Source: CAD feature listing. Evaluate the final solid. Frame: model axes, mm. A direction names the side the tool comes from. Round coordinates to 2 decimals unless told otherwise and drop trailing zeros. Order: outer loops, then holes, each group sorted by start corner. A loop starts at its lowest first (then second) coordinate and runs counter-clockwise, first axis right, second up. Notation, with made-up numbers: (-2, -35.5) - (44, -35.5) arc R22 cw to (44, -28.5) - close; hole circle Ø2 at (-23.75, -37.75). An arc over 180 degrees is marked (long way). Use one line per item in the form item = value. Start each with the question number.
Q1. Cut plane D-D, the plane y = 5.75. Give the number of separate pieces and of enclosed holes in the cut face, and give its area (3 significant figures).
Q2. Ray query, line 1 (X direction, y = 7.75, z = 2.75); line 2 (Y direction, x = -22, z = 3); line 3 (X direction, y = 3.5, z = -12). Return the intervals inside material, ascending. Write a range as [from, to].
Q3. Draft query along X for faces 4 (the flat face through (-9, 3, -6.81)), 5 (the flat face through (-6.36, 3.94, 5.27)), 6 (the cylindrical face through (-21.13, 3.94, -10.83)). Return one class per face: released by +X, released by -X, zero draft, split by the parting line, or undercut.
Q4. Pin query (flat end, axial travel): pin 1 Ø2.5 at (x, y) = (-15, 3.5) entering from +Z; pin 2 Ø4 at (x, z) = (-7, -11.5) entering from -Y; pin 3 Ø0.8 at (x, y) = (0, 3.5) entering from +Z. Return the tip coordinate at first contact, or that it passes through.
Q5. Cut plane B-B, the plane x = 0. Return the cut outline in (y, z) (3 decimals).
Q6. Cut plane C-C, the plane y = 3.75. Return the cut outline in (x, z) (1 decimal), and give its area (3 significant figures).
Q7. Set-up query: faces 1 (the flat face through (0, 4, -0.925)), 2 (the flat face through (-10, 8, -6)), 3 (the flat face through (-20, 5.4, -3)). Return all of +Z, -Z, +X, -X, +Y, -Y with unobstructed straight access to the full face (end or side cutting, diameter ignored); none if empty.
Q8. Cut plane A-A, the plane z = -11. Return the cut outline in (x, y).
Autodesk Inventor part; units mm, degrees
ref_plane "YZ Plane" through (0, 0, 0) normal (1, 0, 0) x (0, 1, 0)
ref_plane "XZ Plane" through (0, 0, 0) normal (0, 1, 0) x (-1, 0, 0)
ref_plane "XY Plane" through (0, 0, 0) normal (0, 0, 1) x (1, 0, 0)
sketch "Sketch1" plane through (0, 0, 0) normal (0, 1, 0) x (-1, 0, 0)
  arc A0 (1.2748, -0.925) -> (-1.2748, -0.925) centre (0, 0) ccw
  line L0 (1.2748, -0.925) -> (-1.2748, -0.925)
  arc A1 (-0.8639, 3.4691) -> (-3.3372, -1.2821) centre (0, 0) ccw
  line L1 (-0.8639, 3.4691) -> (21.9124, 9.141)
  line L2 (-3.3372, -1.2821) -> (5.0806, -23.1927)
  arc A2 (5.0806, -23.1927) -> (21.9124, 9.141) centre (0, 0) ccw
  circle A3 centre (16.2426, 0) radius 4.075
  circle A4 centre (9.3164, -13.3052) radius 4.075
  circle A5 centre (16.2426, 0) radius 7.5 construction
  circle A6 centre (9.3164, -13.3052) radius 7.5 construction
  line L3 (0, 0) -> (16.2426, 0) construction
  line L4 (0, 0) -> (9.3164, -13.3052) construction
  line L5 (12.4926, -6.4952) -> (8.7426, 0)
  line L6 (8.7426, 0) -> (12.4926, 6.4952)
  line L7 (12.4926, 6.4952) -> (19.9926, 6.4952)
  line L8 (19.9926, 6.4952) -> (23.7426, 0)
  line L9 (23.7426, 0) -> (19.9926, -6.4952)
  line L10 (19.9926, -6.4952) -> (12.4926, -6.4952)
  line L11 (16.8164, -13.3052) -> (13.0664, -19.8004)
  line L12 (13.0664, -19.8004) -> (5.5664, -19.8004)
  line L13 (5.5664, -19.8004) -> (1.8164, -13.3052)
  line L14 (1.8164, -13.3052) -> (5.5664, -6.81)
  line L15 (5.5664, -6.81) -> (13.0664, -6.81)
  line L16 (13.0664, -6.81) -> (16.8164, -13.3052)
  dimension "d5" = 15
  dimension "d6" = 15
  dimension "d0" = 3.15
  dimension "d1" = 2.5
  dimension "d2" = 2
  dimension "d3" = 8.15
  dimension "d4" = 8.15
  dimension "d7" = 55
extrude "Extrusion1" add sketch "Sketch1" along normal blind 8 contours L9 L10 L5 L6 L7 L8 | L1 A2 L2 A1 | L11 L12 L13 L14 L15 L16
fillet "Fillet1" radius 8 2 edges at (-21.9124, 4, 9.141) (-5.0806, 4, -23.1927)
extrude "Extrusion2" cut sketch "Sketch1" along normal blind 5.4 contours L9 L10 L5 L6 L7 L8 | L11 L12 L13 L14 L15 L16
sketch "Sketch2" plane through (0, 0, 0) normal (0, -1, 0) x (1, 0, 0)
  arc A0 (-12.8561, -19.8004) -> (-6.2416, -19.8004) centre (-9.5488, -12.516) ccw
  line L0 (-6.2416, -19.8004) -> (-12.8561, -19.8004)
  arc A1 (-12.8561, -19.8004) -> (-6.2416, -19.8004) centre (-9.5488, -12.516) ccw
  line L1 (-23.6968, 0.0794) -> (-20.3388, 5.8956)
  arc A2 (-20.3388, 5.8956) -> (-23.6968, 0.0794) centre (-15.7295, -0.6431) ccw
  line L2 (-12.4926, 6.4952) -> (-8.7426, 0)
  line L3 (-12.4926, 6.4952) -> (-12.6949, 6.8456)
  line L4 (-13.7963, 7.1199) -> (0.8639, 3.4691)
  line L5 (-5.5664, -6.81) -> (-1.8164, -13.3052)
  line L6 (-1.8164, -13.3052) -> (-1.4955, -13.861)
  line L7 (3.3372, -1.2821) -> (-2.081, -15.385)
  line L8 (-1.2748, -0.925) -> (1.2748, -0.925)
  arc A3 (1.2748, -0.925) -> (-1.2748, -0.925) centre (0, 0) ccw
  line L9 (-13.1467, -19.6613) -> (-16.8164, -13.3052)
  line L10 (-16.8164, -13.3052) -> (-13.0664, -6.81)
  line L11 (-13.0664, -6.81) -> (-5.5664, -6.81)
  line L12 (-5.5664, -6.81) -> (-1.8164, -13.3052)
  line L13 (-1.8164, -13.3052) -> (-5.2596, -19.2689)
  arc A4 (-5.2596, -19.2689) -> (-2.081, -15.385) centre (-9.5488, -12.516) ccw
  line L14 (3.3372, -1.2821) -> (-2.081, -15.385)
  arc A5 (3.3372, -1.2821) -> (0.8639, 3.4691) centre (0, 0) ccw
  line L15 (-13.7963, 7.1199) -> (0.8639, 3.4691)
  arc A6 (-13.7963, 7.1199) -> (-19.3413, 6.4952) centre (-15.7295, -0.6431) ccw
  line L16 (-19.3413, 6.4952) -> (-12.4926, 6.4952)
  line L17 (-12.4926, 6.4952) -> (-8.7426, 0)
  line L18 (-8.7426, 0) -> (-12.4926, -6.4952)
  line L19 (-12.4926, -6.4952) -> (-19.9926, -6.4952)
  line L20 (-19.9926, -6.4952) -> (-23.7082, -0.0597)
  arc A7 (-23.7082, -0.0597) -> (-23.7228, -0.9698) centre (-15.7295, -0.6431) ccw
  arc A8 (-23.7228, -0.9698) -> (-14.4013, -18.8763) centre (0, 0) ccw
  arc A9 (-14.4013, -18.8763) -> (-13.1467, -19.6613) centre (-9.5488, -12.516) ccw
  point P0 (-2.081, -15.385)
  point P1 (-13.7963, 7.1199)
extrude "Extrusion3" cut sketch "Sketch2" against normal up to surface (5.4 mm away) contours L0 A0 | A2 L1 | L16 A6 L4 L3 | L7 A4 L13 L6 | A3 L8
properties part number "Desbalanceo"
Completed:
q1.separate_pieces = 1
q1.enclosed_holes = 3
q1.area = 441 mm2
q2.line_1 = [-22.97, -19.25], [-13.24, 2.28]
q2.line_2 = [5.4, 8]
q2.line_3 = [-20.49, -16.06], [-2.57, -0.78]
q3.face_4 = undercut
q3.face_5 = released by +X
q3.face_6 = released by -X
q4.pin_1 = -6.5
q4.pin_2 = 5.4
q4.pin_3 = 3.78
q5.outline = (0, -9.968) - (8, -9.968) - (8, -0.925) - (0, -0.925) - close; (0, 1.575) - (8, 1.575) - (8, 3.684) - (0, 3.684) - close
q6.outline = (-23.7, -1) arc R23.7 ccw to (-14.4, -18.9) arc R8 ccw to (-13.1, -19.7) - (-16.8, -13.3) - (-13.1, -6.8) - (-5.6, -6.8) - (-1.8, -13.3) - (-1.5, -13.9) - (3.3, -1.3) arc R3.6 ccw to (0.9, 3.5) - (-12.7, 6.8) - (-12.5, 6.5) - (-8.7, 0) - (-12.5, -6.5) - (-20, -6.5) - (-23.7, -0.1) arc R8 ccw to start; hole (-1.3, -0.9) - (1.3, -0.9) arc R1.6 ccw (long way) to start
q6.area = 238 mm2
q7.face_1 = +Y, -Y
q7.face_2 = +Z, -Z, +X, -X, +Y
q7.face_3 = -Y
q8.outline = (-21.04, 0) - (-15.49, 0) - (-15.49, 5.4) - (-12.68, 5.4) - (-12.68, 8) - (-21.04, 8) - close; (-5.96, 5.4) - (-3.15, 5.4) - (-3.15, 0) - (-0.4, 0) - (-0.4, 8) - (-5.96, 8) - close
